Geometry check sheet. Reference: the model listing, model coordinates, mm. A direction names the side the tool comes from. Round coordinates to 2 decimals unless told otherwise and drop trailing zeros. Loops run counter-clockwise (first coordinate to the right, second up) from the corner with the lowest first, then second, coordinate; pieces in that order, holes last. Notation, with made-up numbers: (83.5, 28.25) - (126.5, 28.25) arc R15 ccw to (126.5, 45.25) - close; hole circle Ø1 at (63, 5). An arc over 180 degrees is marked (long way). Answer in a Markdown table with one row per item. Add a question column.
```python
from build123d import *

# Parameters (mm, degrees)
SKETCH1_W                                        = 42
SKETCH1_H                                        = 42
BOSS_EXTRUDE1_DEPTH                              = 17
SKETCH2_W                                        = 13
SKETCH2_H                                        = 32.7
CUT_EXTRUDE1_DEPTH                               = 49.30836175
F_22_0_22_DIAMETER_HOLE1_D                       = 22
F_22_0_22_DIAMETER_HOLE1_DEPTH                   = 17
F_3_2_3_2_DIAMETER_HOLE1_D                       = 3.2
F_3_2_3_2_DIAMETER_HOLE1_DEPTH                   = 17
F_3_2_3_2_DIAMETER_HOLE2_D                       = 3.2
F_6_0_6_DIAMETER_HOLE1_D                         = 6
F_6_0_6_DIAMETER_HOLE1_DEPTH                     = 42
F_3_0_3_DIAMETER_HOLE1_D                         = 3
F_3_0_3_DIAMETER_HOLE1_DEPTH                     = 42
CBORE_FOR_M3_HEX_HEAD_MACHINE_SCREW1_D           = 3.2
CBORE_FOR_M3_HEX_HEAD_MACHINE_SCREW1_CBORE_D     = 6
CBORE_FOR_M3_HEX_HEAD_MACHINE_SCREW1_CBORE_DEPTH = 2
FILLET1_R                                        = 1
FILLET2_R                                        = 2


with BuildPart() as part:
    # Sketch1 → Boss-Extrude1 (new body)
    with BuildSketch(Plane(origin=(0, 0, -8.5), x_dir=(-1, 0, 0), z_dir=(0, 0, -1))):
        with Locations((3.196772144, -1.303538171)):
            Rectangle(SKETCH1_W, SKETCH1_H)
    extrude(amount=-BOSS_EXTRUDE1_DEPTH)

    # Sketch2 → Cut-Extrude1 (cut, through all)
    with BuildSketch(Plane(origin=(17.803227856, 0, 0), x_dir=(0, 0, -1), z_dir=(1, 0, 0))):
        with Locations((-2, 3.346461829)):
            Rectangle(SKETCH2_W, SKETCH2_H)
    extrude(amount=-CUT_EXTRUDE1_DEPTH, mode=Mode.SUBTRACT)

    # Ø22.0 (22) Diameter Hole1
    with Locations(Plane(origin=(0, 0, -8.5), x_dir=(-1, 0, 0), z_dir=(0, 0, -1))):
        with Locations((3.196772144, -1.303538171)):
            Hole(F_22_0_22_DIAMETER_HOLE1_D / 2, depth=F_22_0_22_DIAMETER_HOLE1_DEPTH)

    # Ø3.2 (3.2) Diameter Hole1
    with Locations(Plane(origin=(0, 0, -8.5), x_dir=(-1, 0, 0), z_dir=(0, 0, -1))):
        with Locations((-12.303227856, 14.196461829)):
            Hole(F_3_2_3_2_DIAMETER_HOLE1_D / 2, depth=F_3_2_3_2_DIAMETER_HOLE1_DEPTH)

    # Ø3.2 (3.2) Diameter Hole2 (through all)
    with Locations(Plane.XY.offset(8.5)):
        with Locations((-18.696772144, -16.803538171), (12.303227856, -16.803538171)):
            Hole(F_3_2_3_2_DIAMETER_HOLE2_D / 2)

    # Ø6.0 (6) Diameter Hole1
    with Locations(Plane(origin=(0, -22.303538171, 0), x_dir=(-1, 0, 0), z_dir=(0, -1, 0))):
        with Locations((-2.303227856, -2)):
            Hole(F_6_0_6_DIAMETER_HOLE1_D / 2, depth=F_6_0_6_DIAMETER_HOLE1_DEPTH)

    # Ø3.0 (3) Diameter Hole1
    with Locations(Plane(origin=(0, -22.303538171, 0), x_dir=(-1, 0, 0), z_dir=(0, -1, 0))):
        with Locations((14.196772144, -2)):
            Hole(F_3_0_3_DIAMETER_HOLE1_D / 2, depth=F_3_0_3_DIAMETER_HOLE1_DEPTH)

    # CBORE for M3 Hex Head Machine Screw1 (through all)
    with Locations(Plane.XY.offset(-4.5)):
        with Locations((-18.696772144, 14.196461829)):
            CounterBoreHole(CBORE_FOR_M3_HEX_HEAD_MACHINE_SCREW1_D / 2, CBORE_FOR_M3_HEX_HEAD_MACHINE_SCREW1_CBORE_D / 2, CBORE_FOR_M3_HEX_HEAD_MACHINE_SCREW1_CBORE_DEPTH)

    # Fillet1
    fillet1_edges = [part.edges().sort_by_distance(p)[0] for p in [
        (-24.196772144, 19.696461829, -6.5),
        (17.803227856, 19.696461829, -6.5),
    ]]
    fillet(fillet1_edges, radius=FILLET1_R)

    # Fillet2
    fillet2_edges = [part.edges().sort_by_distance(p)[0] for p in [
        (17.803227856, -22.303538171, 0),
        (-24.196772144, -22.303538171, 0),
    ]]
    fillet(fillet2_edges, radius=FILLET2_R)


solid = part.part
```
Q1. Release check for a two-part mould opening along Y. For faces 4 (the flat face through (-3, -22.304, 0)), 5 (the cylindrical face through (-21.1, 12.4, -5.5)), 6 (the cylindrical face through (-12.766, -17.588, 1.549)) record: +Y half, -Y half, draft (parallel to the pull), parting line (faces both ways), or undercut.
Q2. Cross-section at D-D, the plane x = 1.5. Enter the section's corners in (y, z), plus the area to 3 significant figures.
Q3. Set-up check for faces 1 (the flat face through (-12, 8, -8.5)), 2 (the flat face through (-17, 13, -6.5)), 3 (the flat face through (-3, 10, -4.5)): record each of +Z, -Z, +X, -X, +Y, -Y from which the full face is reachable in a straight line by a thin tool's end or side.
Q4. Depth check by flat-ended pin: P1, Ø5, axis at x = -18.7, y = 14.2, coming from the -Z side; P2, Ø3, axis at x = 12, y = -7.5, coming from the +Z side; P3, Ø10, axis at x = 5.5, z = 5.5, coming from the +Y side. Enter the tip coordinate at first touch or a pass-through.
Q5. Cross-section at C-C, the plane z = 4.5. Enter the section's corners in (x, y), plus the area to 3 significant figures.
Q6. Scan lines: line 1 (Y direction, x = -18.5, z = -1); line 2 (Z direction, x = -14, y = 14); line 3 (Y direction, x = 1.5, z = -3). Record each from-to range of solid material in increasing order. Write a range as from..to.
Q7. Cross-section at B-B, the plane y = 4. Enter the section's corners in (x, z), plus the area to 3 significant figures.
Q8. Cross-section at A-A, the plane z = 2. Enter the section's corners in (x, y), plus the area to 3 significant figures.
Check sheet entries:
| question | item | result |
|---|---|---|
| 1 | face 4 | -Y half |
| 1 | face 5 | undercut |
| 1 | face 6 | draft |
| 2 | outline | (-22.3, -8.5) - (-11.25, -8.5) - (-11.25, -4.5) - (-13, -4.5) - (-13, -0.89) - (-22.3, -0.89) - close; (-22.3, 4.89) - (-13, 4.89) - (-13, 8.5) - (-22.3, 8.5) - close; (8.64, -8.5) - (19.7, -8.5) - (19.7, -4.5) - (8.64, -4.5) - close |
| 2 | area | 156 mm² |
| 3 | face 1 | -Z, +X, -X, +Y, -Y |
| 3 | face 2 | +Z |
| 3 | face 3 | +Z, +X, -X, +Y |
| 4 | P1 | z = -8.5 |
| 4 | P2 | z = -4.5 |
| 4 | P3 | y = -13 |
| 5 | outline | (-24.2, -20.3) arc R2 ccw to (-22.2, -22.3) - (0.64, -22.3) - (0.64, -13) - (-24.2, -13) - close; (3.96, -22.3) - (15.8, -22.3) arc R2 ccw to (17.8, -20.3) - (17.8, -13) - (3.96, -13) - close; hole circle Ø3.2 at (-18.7, -16.8); hole circle Ø3.2 at (12.3, -16.8) |
| 5 | area | 342 mm² |
| 6 | line 1 | -22.3..-18.39, -15.22..-13 |
| 6 | line 2 | -8.5..-4.5 |
| 6 | line 3 | -22.3..-13 |
| 7 | outline | (-24.2, -8.5) - (-12.83, -8.5) - (-12.83, -4.5) - (-24.2, -4.5) - close; (6.44, -8.5) - (17.8, -8.5) - (17.8, -4.5) - (6.44, -4.5) - close |
| 7 | area | 90.9 mm² |
| 8 | outline | (-24.2, -20.3) arc R2 ccw to (-22.2, -22.3) - (-15.7, -22.3) - (-15.7, -13) - (-24.2, -13) - close; (-12.7, -22.3) - (-0.7, -22.3) - (-0.7, -13) - (-12.7, -13) - close; (5.3, -22.3) - (15.8, -22.3) arc R2 ccw to (17.8, -20.3) - (17.8, -13) - (5.3, -13) - close; hole circle Ø3.2 at (-18.7, -16.8); hole circle Ø3.2 at (12.3, -16.8) |
| 8 | area | 289 mm² |
